from build123d import *

# Parameters (mm, degrees)
SKETCH1_R           = 5.4
BOSS_EXTRUDE1_DEPTH = 34.925
FILLET1_R           = 10


with BuildPart() as part:
    # Sketch1 → Boss-Extrude1 (new body)
    with BuildSketch(Plane.XY):
        Polygon((0, 0), (25.4, 0), (25.4, -76.2), (38.1, -76.2), (38.1, 25), (0, 25), align=None)
        with Locations((25.4, 12.5)):
            Circle(SKETCH1_R, mode=Mode.SUBTRACT)
    extrude(amount=BOSS_EXTRUDE1_DEPTH)

    # Fillet1
    fillet1_edges = [part.edges().sort_by_distance(p)[0] for p in [
        (38.1, 25, 17.4625),
    ]]
    fillet(fillet1_edges, radius=FILLET1_R)


solid = part.part
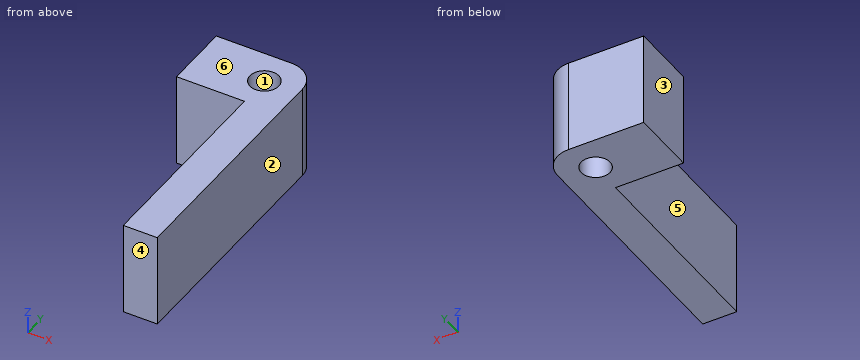
Here's how the part is built. I have some questions about the finished solid (model axes, mm). Face numbers are marked on the shaded views. A direction names the side the tool comes from. Round coordinates to 2 decimals unless told otherwise and drop trailing zeros. Order: outer loops, then holes, each group sorted by start corner. A loop starts at its lowest first (then second) coordinate and runs counter-clockwise, first axis right, second up. Notation, with made-up numbers: M 54,-16 L 60,-16 A18 cw 60,1 Z; hole C 80.5,56.25 d7. An arc over 180 degrees is marked long. Return JSON: item names as keys, results as strings. Group by question number.
1. If we section it at B-B on z = 5: List the corners of the cut face in (x, y) for me, then the cut area to 3 significant figures.
2. If we section it at A-A on y = 12.5: List the corners of the cut face in (x, z) for me (3 decimals).
3. I'm going to push flat-ended pins straight in: pin 1 Ø4 at (y, z) = (-4, 26) entering from -X; pin 2 Ø20.5 at (x, z) = (10, 13.5) entering from -Y. Where does each tip first touch, or does it pass through?
4. If we section it at C-C on x = 22: List the corners of the cut face in (y, z) for me (3 decimals), then the cut area to 3 significant figures.
5. On a 3-axis mill with a long thin cutter (end or side, diameter ignored), from which of +Z, -Z, +X, -X, +Y, -Y can I reach the whole of each face in a straight line? I mean the marked faces 5 and 6. Say none if no direction works.
6. If we section it at D-D on y = -26: List the corners of the cut face in (x, z) for me (3 decimals), then the cut area to 3 significant figures.
7. If we mould it in two halves opening along X, with no side actions, what happens to the marked faces 1, 2, 3 and 4? For each: pulls with the +X half, pulls with the -X half, needs draft (parallel to the pull), parting line crosses it, or undercut.
8. Please list where these lines run through material, in increasing order: probe 1 along X at (y, z) = (12, 25); probe 2 along Y at (x, z) = (25, 14); probe 3 along Y at (x, z) = (6.5, 2.5).
Reply:
{
 "1": {"outline": "M 0,0 L 25.4,0 L 25.4,-76.2 L 38.1,-76.2 L 38.1,15 A10 ccw 28.1,25 L 0,25 Z; hole C 25.4,12.5 d10.8", "area": "1,810 mm^2"},
 "2": {"outline": "M 0,0 L 20,0 L 20,34.925 L 0,34.925 Z; M 30.8,0 L 38.1,0 L 38.1,34.925 L 30.8,34.925 Z"},
 "3": {"pin 1": "x = 25.4", "pin 2": "y = 0"},
 "4": {"outline": "M 0,0 L 8.305,0 L 8.305,34.925 L 0,34.925 Z; M 16.695,0 L 25,0 L 25,34.925 L 16.695,34.925 Z", "area": "580 mm^2"},
 "5": {"face 5": "+Z, -Z, -X, -Y", "face 6": "+Z, +X, -X, +Y, -Y"},
 "6": {"outline": "M 25.4,0 L 38.1,0 L 38.1,34.925 L 25.4,34.925 Z", "area": "444 mm^2"},
 "7": {"face 1": "undercut", "face 2": "pulls with the +X half", "face 3": "pulls with the -X half", "face 4": "needs draft"},
 "8": {"probe 1": "0 to 20.02, 30.78 to 38.1", "probe 2": "0 to 7.11, 17.89 to 25", "probe 3": "0 to 25"}
}
